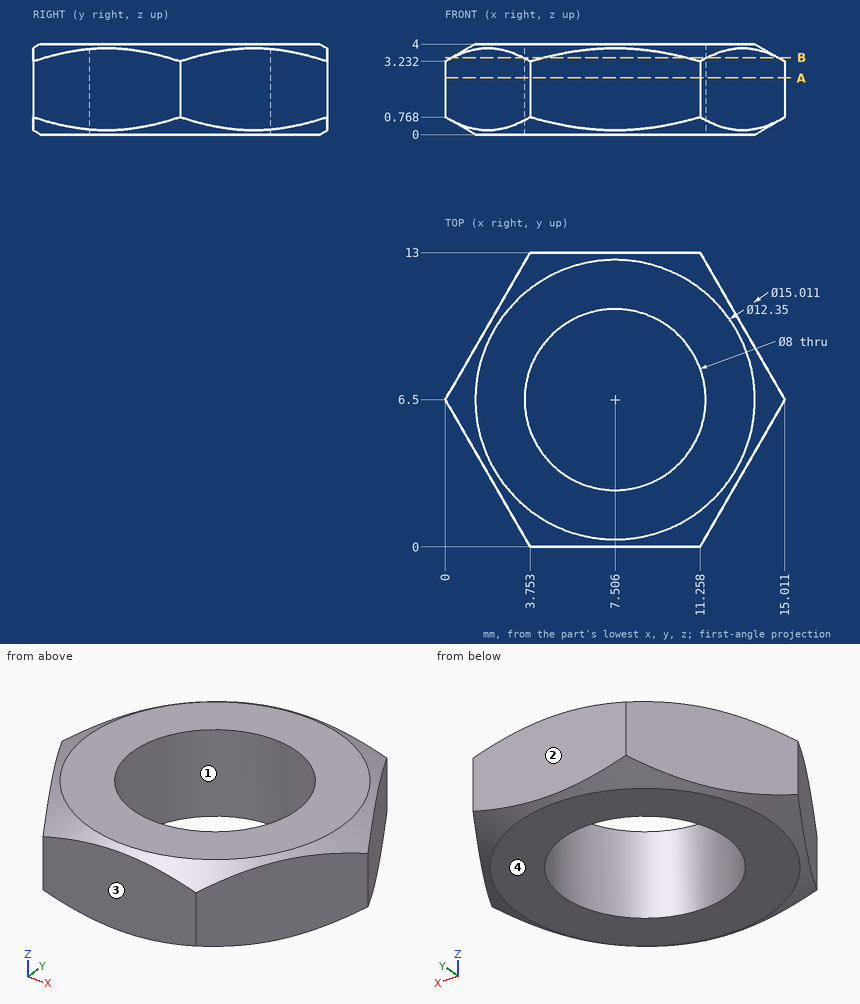
Geometry check sheet. Reference: drawing and pictorial views, mm from the part's lowest x, y, z. Give positions to 0.01 mm unless a question says otherwise; leave off trailing zeros. Loops run counter-clockwise (first coordinate to the right, second up) from the corner with the lowest first, then second, coordinate; pieces in that order, holes last.
1. Section check A-A, the plane z = 2.5. Enter the section's corners in (x, y) (1 decimal).
2. Section check B-B, the plane z = 3.4. Enter the section's corners in (x, y) (1 decimal).
3. Thickness scan on line 1 (Y direction, x = 7.5, z = 0.5); line 2 (X direction, y = 8.75, z = 1.3); line 3 (Y direction, x = 10, z = 2.1) (1 decimal). Record the ranges inside material, lowest first.
4. Mould release check, pull along Y, two halves, no side actions. Record for the marked faces 1, 2, 3 and 4: released by +Y, released by -Y, zero draft, split by the parting line, or undercut.
Geometry says:
1. outline: (0, 6.5) - (3.8, 0) - (11.3, 0) - (15, 6.5) - (11.3, 13) - (3.8, 13) - close; hole circle Ø8 at (7.5, 6.5)
2. outline: (0.3, 6) - (3.4, 0.5) arc R7.2 ccw to (4.4, 0) - (10.6, 0) arc R7.2 ccw to (11.6, 0.5) - (14.7, 6) arc R7.2 ccw to (14.7, 7) - (11.6, 12.5) arc R7.2 ccw to (10.6, 13) - (4.4, 13) arc R7.2 ccw to (3.4, 12.5) - (0.3, 7) arc R7.2 ccw to start; hole circle Ø8 at (7.5, 6.5)
3. line 1: y = 0 to 2.5, 10.5 to 13
3. line 2: x = 1.3 to 4.2, 10.81 to 13.71
3. line 3: y = 0 to 3.4, 9.6 to 13
4. face 1: undercut
4. face 2: released by +Y
4. face 3: released by -Y
4. face 4: zero draft
